Autodesk Inventor part; units mm, degrees
ref_plane "YZ Plane" through (0, 0, 0) normal (1, 0, 0) x (0, 1, 0)
ref_plane "XZ Plane" through (0, 0, 0) normal (0, 1, 0) x (-1, 0, 0)
ref_plane "XY Plane" through (0, 0, 0) normal (0, 0, 1) x (1, 0, 0)
sketch "Esquisse4" plane through (0, 0, 0) normal (0, 1, 0) x (-1, 0, 0)
  circle A0 centre (0, 0) radius 2.25
  circle A1 centre (0, 0) radius 4
  dimension "d6" = 4.5
  dimension "d7" = 8
extrude "Extrusion2" add sketch "Esquisse4" along normal blind 8
sketch "Esquisse5" plane through (0, 8, 0) normal (0, 1, 0) x (1, 0, 0)
  circle A0 centre (0, 0) radius 4
  circle A1 centre (0, 0) radius 88.9
  spline S0 degree 3 poles (-88.9, 0) (-96.1137, 15.1507) (-22.3547, 20.9921) (-3.3072, 2.25) knots 0 0 0 0 1 1 1 1
  spline S1 degree 2 poles (-88.9, 0) (-58.1385, -7.7753) (-3.873, -1) knots 0 0 0 1 1 1
  point P0 (-86.0001, 7)
  point P1 (-47, 14)
  point P2 (-58, -4)
  dimension "d10" = 177.8
extrude "Extrusion3" add sketch "Esquisse5" against normal blind 2 contours A0 S1 A1 S0 | A1 S0 picked at (-43.854, 2.0054)
pattern_circular "Réseau circulaire1" count 2 over 360 about axis through (0, 0, 0) along (0, -1, 0) of "Extrusion3"
properties part number "Helice 7x3" material "Plastique ABS"
Design review of the part built by this model. Coordinates are the model's own, in mm. Give positions to 0.01 mm unless a question says otherwise; leave off trailing zeros. Write each loop counter-clockwise with the first axis right and the second up, starting at its lowest first coordinate (ties: lowest second). Pieces come first, ordered by that corner, then holes. Notation, with made-up numbers: M 13,-28 L 32,-28 A25 cw 32,-11 Z; hole C -7.75,-37.5 d1. An arc over 180 degrees is marked long. Answer as a JSON object with one key per item and string values. Group by question number.
1) Clearance check with flat-ended pins moving along their axes: pin 1 Ø3 at (y, z) = (2, -2.5) entering from -X; pin 2 Ø4 at (y, z) = (6, 9.5) entering from -X; pin 3 Ø2 at (x, y) = (49.5, 6.5) entering from +Z. State where each tip first meets the part, or that it passes through.
2) We need section B-B (y = 3). Give the boundary of the cut face in (x, z), and give its area (3 significant figures).
3) Mouldability with a two-part tool opening along X and no side actions: class faces 1 (the face through (0.29, 3.94, -2.23)), 2 (the face through (0, 8, 3)) as released by +X, released by -X, zero draft, split by the parting line, or undercut.
4) For line 1 along Z through (x, y) = (0, 3.25); line 2 along Y through (x, z) = (-74, 1.75); line 3 along X through (y, z) = (3.5, 1.5), list the stretches that pass through material, from the lowest coordinate up.
5) We need section A-A (x = 0). Give the boundary of the cut face in (y, z), and give its area (3 significant figures).
Answer key:
{
 "1": {"pin 1": "stops at x = -3.87", "pin 2": "stops at x = 11.26", "pin 3": "stops at z = 14.01"},
 "2": {"outline": "C 0,0 d8; hole C 0,0 d4.5", "area": "34.4 mm²"},
 "3": {"face 1": "undercut", "face 2": "zero draft"},
 "4": {"line 1": "z = -4 to -2.25, 2.25 to 4", "line 2": "y = 6 to 8", "line 3": "x = -3.71 to -1.68, 1.68 to 3.71"},
 "5": {"outline": "M 0,-4 L 8,-4 L 8,-2.25 L 0,-2.25 Z; M 0,2.25 L 8,2.25 L 8,4 L 0,4 Z", "area": "28.0 mm²"}
}
